For this review, take the finished solid that the model builds, in its own axes (mm). A direction names the side the tool comes from. Give positions to 0.01 mm unless a question says otherwise; leave off trailing zeros. Write each loop counter-clockwise with the first axis right and the second up, starting at its lowest first coordinate (ties: lowest second). Pieces come first, ordered by that corner, then holes.
1) Draft analysis for pull direction Z (two halves, no side actions). For faces 1 (the face through (6.549, -44.643, 38.825)), 2 (the face through (6.55, -34.88, 1.08)), 3 (the face through (11, 3, -20)), 4 (the face through (12, 10, 10)), state which applies: pulls with the +Z half, pulls with the -Z half, needs draft (parallel to the pull), parting line crosses it, or undercut.
2) We need section D-D on z = 30. Give the boundary of the cut face in (x, y), and give its area (3 significant figures).
3) We need section B-B on y = 1.5. Give the boundary of the cut face in (x, z).
4) Wall thickness on line 1 along X through (y, z) = (2.75, -10); line 2 along X through (y, z) = (-43, 38.5); line 3 along Y through (x, z) = (10.75, 19.5): over which ranges is each line inside the solid? List them lowest first.
5) For P1, Ø3.5, axis at x = 10, y = 3.5, coming from the -Z side; P2, Ø6, axis at x = 15.5, z = -10, coming from the +Y side; P3, Ø3, axis at y = -32, z = 40, coming from the +X side, all flat-tipped, find the tip position at first contact; note any pin that passes through.
6) We need section A-A on z = -10. Give the boundary of the cut face in (x, y).
7) Machinability: for faces 5 (the face through (6, 0, -21)), 6 (the face through (12, 10, -10)), 7 (the face through (11, 3, 20)), 8 (the face through (15, 0, 0)), which of the approach directions +Z, -Z, +X, -X, +Y, -Y give a long, thin tool a straight path to every point of the face, cutting with its end or side? Answer none if there is none.
from build123d import *

# Parameters (mm, degrees)
CROQUIS1_W              = 40
CROQUIS1_H              = 40
SALIENTE_EXTRUIR1_DEPTH = 7
CROQUIS3_W              = 5.6
CROQUIS3_H              = 5.7
SALIENTE_EXTRUIR3_DEPTH = 40
CROQUIS19_W             = 8
CROQUIS19_H             = 40
CORTAR_EXTRUIR5_DEPTH   = 5.7
CROQUIS20_R             = 2.5
CORTAR_EXTRUIR6_DEPTH   = 7
CROQUIS21_W             = 7
CROQUIS21_H             = 72
SALIENTE_EXTRUIR4_DEPTH = 50
CROQUIS22_R             = 5
CORTAR_EXTRUIR7_DEPTH   = 7
CROQUIS25_R             = 4.25
CORTAR_EXTRUIR8_DEPTH   = 3.5
REDONDEO1_R             = 30
REDONDEO2_R             = 30
CROQUIS29_W             = 103.753326912
CROQUIS29_H             = 179.412983462
CORTAR_EXTRUIR9_DEPTH   = 23


# Some blends are built 0.0001 mm under size
with BuildPart() as part:
    # Croquis1 → Saliente-Extruir1 (new body)
    with BuildSketch(Plane(origin=(0, 0, 0), x_dir=(1, 0, 0), z_dir=(0, 1, 0))):
        Rectangle(CROQUIS1_W, CROQUIS1_H)
    extrude(amount=SALIENTE_EXTRUIR1_DEPTH)

    # Croquis3 → Saliente-Extruir3 (add)
    with BuildSketch(Plane.ZY.offset(20)):
        with Locations((10, 9.85)):
            Rectangle(CROQUIS3_W, CROQUIS3_H)
        with Locations((-10, 9.85)):
            Rectangle(CROQUIS3_W, CROQUIS3_H)
    extrude(amount=-SALIENTE_EXTRUIR3_DEPTH)

    # Croquis19 → Cortar-Extruir5 (cut)
    with BuildSketch(Plane(origin=(0, 12.7, 0), x_dir=(1, 0, 0), z_dir=(0, 1, 0))):
        with Locations((-16, 0)):
            Rectangle(CROQUIS19_W, CROQUIS19_H)
        with Locations((16, 0)):
            Rectangle(CROQUIS19_W, CROQUIS19_H)
    extrude(amount=-CORTAR_EXTRUIR5_DEPTH, mode=Mode.SUBTRACT)

    # Croquis20 → Cortar-Extruir6 (cut)
    with BuildSketch(Plane(origin=(0, 7, 0), x_dir=(1, 0, 0), z_dir=(0, 1, 0))):
        with Locations(Location((-15.5, 10, 0), (0, 0, 270))):
            Circle(CROQUIS20_R)
        with Locations(Location((15.5, 10, 0), (0, 0, 270))):
            Circle(CROQUIS20_R)
        with Locations(Location((15.5, -10, 0), (0, 0, 270))):
            Circle(CROQUIS20_R)
        with Locations(Location((-15.5, -10, 0), (0, 0, 270))):
            Circle(CROQUIS20_R)
    extrude(amount=-CORTAR_EXTRUIR6_DEPTH, mode=Mode.SUBTRACT)

    # Croquis21 → Saliente-Extruir4 (add)
    with BuildSketch(Plane.XZ):
        with Locations((6.5, 14)):
            Rectangle(CROQUIS21_W, CROQUIS21_H)
    extrude(amount=SALIENTE_EXTRUIR4_DEPTH)

    # Croquis22 → Cortar-Extruir7 (cut)
    with BuildSketch(Plane(origin=(10, 0, 0), x_dir=(0, 0, -1), z_dir=(1, 0, 0))):
        with Locations((0, -30)):
            Circle(CROQUIS22_R)
    extrude(amount=-CORTAR_EXTRUIR7_DEPTH, mode=Mode.SUBTRACT)

    # Croquis25 → Cortar-Extruir8 (cut)
    with BuildSketch(Plane(origin=(10, 0, 0), x_dir=(0, 0, -1), z_dir=(1, 0, 0))):
        with Locations((-30, -30)):
            Circle(CROQUIS25_R)
    extrude(amount=-CORTAR_EXTRUIR8_DEPTH, mode=Mode.SUBTRACT)

    # Redondeo1
    redondeo1_edges = [part.edges().sort_by_distance(p)[0] for p in [
        (6.5, 0, 50),
    ]]
    fillet(redondeo1_edges, radius=REDONDEO1_R - 0.0001)  # a hair under: the kernel refuses the full size

    # Redondeo2
    # the kernel refuses this fillet: 30 mm, written as the material it takes off along each edge
    with BuildSketch(Plane(origin=(80.710766507, -50, 50), x_dir=(0, 1, 0), z_dir=(-1, 0, 0))) as redondeo2_piece_1:
        with BuildLine():
            CenterArc((30, 28.284306603), REDONDEO2_R, 180, 70.528981937)
            Line((0, 28.284306603), (-0.6, 28.284306603))
            Line((-0.6, 28.284306603), (-0.6, 0))
            Line((-0.6, 0), (0, -0.6))
            ThreePointArc((0, -0.6), (10.00005, -0.6), (19.800102, -0.565686132))
            Line((19.800102, -0.565686132), (20.0001, 0))
        make_face()
    extrude(amount=148.421533013, mode=Mode.SUBTRACT)

    # Croquis29 → Cortar-Extruir9 (cut)
    with BuildSketch(Plane.ZY.offset(20)):
        Rectangle(CROQUIS29_W, CROQUIS29_H)
    extrude(amount=-CORTAR_EXTRUIR9_DEPTH, mode=Mode.SUBTRACT)


solid = part.part
Results list:
1. face 1: pulls with the +Z half
1. face 2: undercut
1. face 3: pulls with the -Z half
1. face 4: needs draft
2. outline: (3, -48.83) - (10, -48.83) - (10, -34.25) - (6.5, -34.25) - (6.5, -25.75) - (10, -25.75) - (10, -1.72) - (3, -1.72) - close
2. area: 300 mm2
3. outline: (3, -20) - (20, -20) - (20, 20) - (3, 20) - close; hole circle Ø5 at (15.5, -10); hole circle Ø5 at (15.5, 10)
4. line 1: x = 3 to 13, 18 to 20
4. line 2: x = 3 to 10
4. line 3: y = 0 to 7
5. P1: stops at z = -20
5. P2: stops at y = 7
5. P3: stops at x = 10
6. outline: (3, -50) - (10, -50) - (10, 0) - (13, 0) - (13, 7) - (12, 7) - (12, 12.7) - (3, 12.7) - close; (18, 0) - (20, 0) - (20, 7) - (18, 7) - close
7. face 5: -Z, +X, -X, +Y
7. face 6: +Z, -Z, +X, +Y
7. face 7: +Z, +X, -X, +Y
7. face 8: +Z, -Z, +X, -Y
